from build123d import *

# Parameters (mm, degrees)
PAD021_DEPTH    = 1046
THICKNESS001_T  = -18
SKETCH040_W     = 50
SKETCH040_H     = 50
SKETCH040_W_2   = 100
POCKET001_DEPTH = 18
SKETCH048_W     = 36
SKETCH048_H     = 18
PAD028_DEPTH    = 1464
SKETCH049_W     = 54
SKETCH049_H     = 18
PAD029_DEPTH    = 1010


with BuildPart() as part:
    # Sketch039 → Pad021 (new body)
    with BuildSketch(Plane.YZ):
        Polygon((0, 0), (0, 150), (870, 450), (1500, 450), (1500, 0), align=None)
    extrude(amount=PAD021_DEPTH)

    # Thickness001
    thickness001_openings = [part.faces().sort_by_distance(p)[0] for p in [
        (523, 750, 0),
    ]]
    offset(amount=THICKNESS001_T, openings=thickness001_openings)

    # Sketch040 → Pocket001 (cut)
    with BuildSketch(Plane(origin=(0, 1500, 0), x_dir=(-1, 0, 0), z_dir=(0, 1, 0))):
        with Locations((-898, 25)):
            Rectangle(SKETCH040_W, SKETCH040_H)
        with Locations((-148, 25)):
            Rectangle(SKETCH040_W, SKETCH040_H)
        with Locations((-523, 25)):
            Rectangle(SKETCH040_W_2, SKETCH040_H)
    extrude(amount=-POCKET001_DEPTH, mode=Mode.SUBTRACT)

    # Sketch048 → Pad028 (new body)
    with BuildSketch(Plane(origin=(0, 18, 0), x_dir=(-1, 0, 0), z_dir=(0, 1, 0))):
        with Locations((-1010, 59)):
            Rectangle(SKETCH048_W, SKETCH048_H)
        with Locations((-36, 59)):
            Rectangle(SKETCH048_W, SKETCH048_H)
    extrude(amount=PAD028_DEPTH)

    # Sketch049 → Pad029 (new body)
    with BuildSketch(Plane(origin=(0, 0, 0), x_dir=(0, -1, 0), z_dir=(-1, 0, 0))):
        with Locations((-45, 59)):
            Rectangle(SKETCH049_W, SKETCH049_H)
        with Locations((-1455, 59)):
            Rectangle(SKETCH049_W, SKETCH049_H)
    extrude(amount=-PAD029_DEPTH)


solid = part.part
The model under review builds one solid part; all positions refer to its coordinate system, in mm. A direction names the side the tool comes from. Give positions to 0.01 mm unless a question says otherwise; leave off trailing zeros. Loops run counter-clockwise (first coordinate to the right, second up) from the corner with the lowest first, then second, coordinate; pieces in that order, holes last. Notation, with made-up numbers: (63.5, -30) -> (89.5, -30) arc R29 cw to (89.5, 0) -> close; hole circle Ø1 at (76.5, 30.25). An arc over 180 degrees is marked (long way). Put each result on its own line as item: value. Start each with the question number.
1. For faces 1 (the face through (1028, 760, 25)), 2 (the face through (516, 1500, 228)), 3 (the face through (1028, 923, 212)), list the 3-axis set-ups (+Z, -Z, +X, -X, +Y, -Y) from which the entire face can be reached by the end or side of a thin tool; tool diameter is ignored.
2. We need section D-D on z = 238. State the section outline as (x, y) points, then the cut area to 3 significant figures.
3. We need section B-B on x = 751. State the section outline as (y, z) points.
4. Mouldability with a two-part tool opening along Y and no side actions: class faces 4 (the face through (516, 1173, 432)), 5 (the face through (516, 1181, 450)), 6 (the face through (515.68, 428.91, 297.9)) as released by +Y, released by -Y, zero draft, split by the parting line, or undercut.
5. Clearance check with flat-ended pins moving along their axes: P1, Ø12, axis at x = 659, y = 943.5, coming from the -Z side; P2, Ø1.5, axis at x = 106.5, y = 187.5, coming from the -Z side. State where each tip first meets the part, or that it passes through.
6. We need section C-C on y = 1350.5. State the section outline as (x, z) points.
7. Wall thickness on probe 1 along X at (y, z) = (1255, 113); probe 2 along Y at (x, z) = (983, 87); probe 3 along X at (y, z) = (208.5, 67): over which ranges is each line inside the solid? List them lowest first.
8. We need section A-A on z = 107. State the section outline as (x, y) points, then the cut area to 3 significant figures.
Determined:
1. face 1: -Z
1. face 2: +Z, -Z, +X, -X, +Y
1. face 3: none
2. outline: (0, 255.2) -> (1046, 255.2) -> (1046, 1500) -> (0, 1500) -> close; hole (18, 310.42) -> (1028, 310.42) -> (1028, 1482) -> (18, 1482) -> close
2. area: 119,000 mm^2
3. outline: (0, 0) -> (18, 0) -> (18, 50) -> (72, 50) -> (72, 68) -> (18, 68) -> (18, 137.17) -> (873.02, 432) -> (1482, 432) -> (1482, 68) -> (1428, 68) -> (1428, 50) -> (1482, 50) -> (1482, 0) -> (1500, 0) -> (1500, 450) -> (870, 450) -> (0, 150) -> close
4. face 4: undercut
4. face 5: zero draft
4. face 6: released by -Y
5. P1: z = 432
5. P2: z = 195.36
6. outline: (0, 0) -> (18, 0) -> (18, 50) -> (54, 50) -> (54, 68) -> (18, 68) -> (18, 432) -> (1028, 432) -> (1028, 68) -> (992, 68) -> (992, 50) -> (1028, 50) -> (1028, 0) -> (1046, 0) -> (1046, 450) -> (0, 450) -> close
7. probe 1: 0 to 18, 1028 to 1046
7. probe 2: 0 to 18, 1482 to 1500
7. probe 3: 0 to 54, 992 to 1046
8. outline: (0, 0) -> (1046, 0) -> (1046, 1500) -> (0, 1500) -> close; hole (18, 18) -> (1028, 18) -> (1028, 1482) -> (18, 1482) -> close
8. area: 90,400 mm^2
